Design review of the part shown in the three views and the two pictorial views. Dimensions are in mm from the part's minimum x, y and z. Coordinates: 2 decimals unless noted, no trailing zeros. Write each loop counter-clockwise with the first axis right and the second up, starting at its lowest first coordinate (ties: lowest second). Pieces come first, ordered by that corner, then holes. Notation, with made-up numbers: (43, 3.5) - (79, 3.5) arc R19 cw to (79, 23.5) - close; hole circle Ø1 at (66, 37.25). An arc over 180 degrees is marked (long way). Write each question's results on one line, items separated by ' | '.
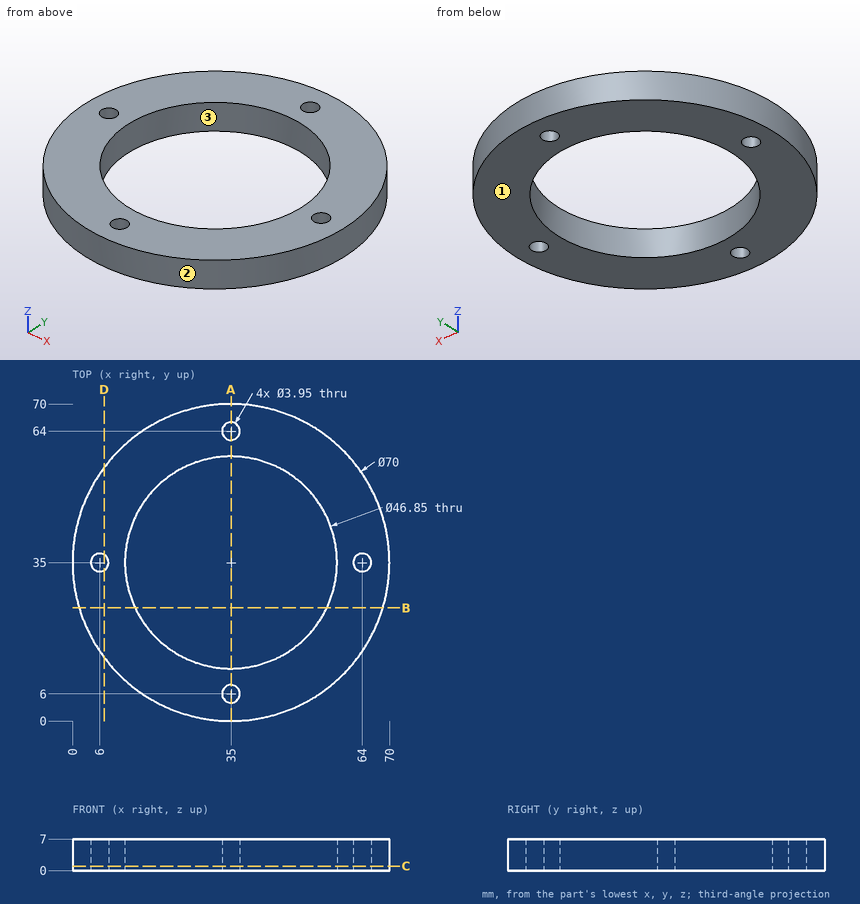
Q1. Take a section at C-C on z = 1. State the section outline as (x, y) points (3 decimals).
Results found:
outline: circle Ø70 at (35, 35); hole circle Ø3.95 at (6, 35); hole circle Ø46.85 at (35, 35); hole circle Ø3.95 at (35, 6); hole circle Ø3.95 at (35, 64); hole circle Ø3.95 at (64, 35)
Q2. Take a section at B-B on y = 25. State the section outline as (x, z) points.
Results found:
outline: (1.46, 0) - (13.82, 0) - (13.82, 7) - (1.46, 7) - close; (56.18, 0) - (68.54, 0) - (68.54, 7) - (56.18, 7) - close
Q3. Wall thickness on line 1 along Y through (x, z) = (35, 3) (3 decimals); line 2 along X through (y, z) = (36, 4); line 3 along Y through (x, z) = (22.5, 2.75): over which ranges is each line inside the solid? List them lowest first. Write a range as from..to.
Results found:
line 1: 0..4.025, 7.975..11.575, 58.425..62.025, 65.975..70 | line 2: 0.01..4.3, 7.7..11.6, 58.4..62.3, 65.7..69.99 | line 3: 2.31..15.19, 54.81..67.69
Q4. For pin 1 (2.5 mm diameter, centred on x = 6, y = 35, fed in from +Z); pin 2 (1.5 mm diameter, centred on y = 52, z = 2.5, fed in from -X); pin 3 (1 mm diameter, centred on x = 54.5, z = 5.5, fed in from -Y); pin 4 (1 mm diameter, centred on x = 10, z = 3, fed in from -Y) (3 decimals), all flat-tipped, find the tip position at first contact; note any pin that passes through.
Results found:
pin 1: through | pin 2: x = 4 | pin 3: y = 5.61 | pin 4: y = 10.005
Q5. Mouldability with a two-part tool opening along X and no side actions: class the marked faces 1, 2 and 3 as pulls with the +X half, pulls with the -X half, needs draft (parallel to the pull), parting line crosses it, or undercut.
Results found:
face 1: needs draft | face 2: parting line crosses it | face 3: undercut
Q6. Take a section at D-D on x = 7. State the section outline as (y, z) points.
Results found:
outline: (14, 0) - (33.3, 0) - (33.3, 7) - (14, 7) - close; (36.7, 0) - (56, 0) - (56, 7) - (36.7, 7) - close
Q7. Take a section at A-A on x = 35. State the section outline as (y, z) points (3 decimals), plus the area to 3 significant figures.
Results found:
outline: (0, 0) - (4.025, 0) - (4.025, 7) - (0, 7) - close; (7.975, 0) - (11.575, 0) - (11.575, 7) - (7.975, 7) - close; (58.425, 0) - (62.025, 0) - (62.025, 7) - (58.425, 7) - close; (65.975, 0) - (70, 0) - (70, 7) - (65.975, 7) - close | area: 107 mm2
